The listing builds one solid part. Answer for the finished solid, in the listing's coordinates (mm). Face numbers are marked on the shaded views. Give positions to 0.01 mm unless a question says otherwise; leave off trailing zeros. Order: outer loops, then holes, each group sorted by start corner. A loop starts at its lowest first (then second) coordinate and runs counter-clockwise, first axis right, second up.
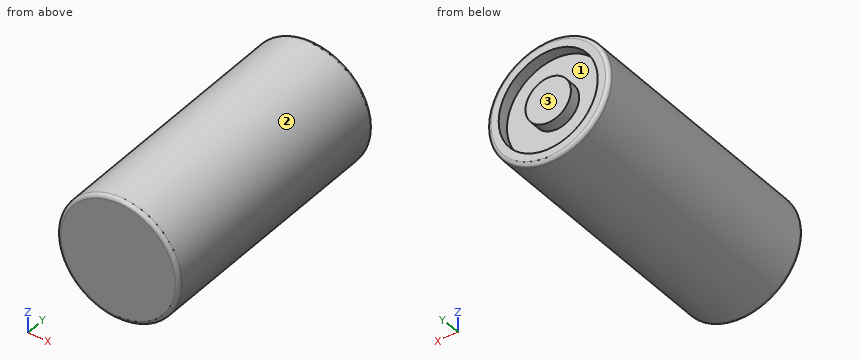
```python
from build123d import *

# Parameters (mm, degrees)
SKETCH_1_R          = 16.1
EXTRUDE_1_DEPTH     = 70.6
SKETCH_3_R          = 13.073776485
SKETCH_3_R_2        = 6
CUT_EXTRUDE_1_DEPTH = 3
FILLET_1_R          = 1
FILLET_2_R          = 1


with BuildPart() as part:
    # 草图1 → 凸台-拉伸1 (new body)
    with BuildSketch(Plane(origin=(0, 0, 0), x_dir=(1, 0, 0), z_dir=(0, 1, 0))):
        Circle(SKETCH_1_R)
    extrude(amount=EXTRUDE_1_DEPTH)

    # 草图3 → 切除-拉伸1 (cut)
    with BuildSketch(Plane(origin=(0, 70.6, 0), x_dir=(1, 0, 0), z_dir=(0, 1, 0))):
        Circle(SKETCH_3_R)
        Circle(SKETCH_3_R_2, mode=Mode.SUBTRACT)
    extrude(amount=-CUT_EXTRUDE_1_DEPTH, mode=Mode.SUBTRACT)

    # 圆角1
    fillet_1_edges = [part.edges().sort_by_distance(p)[0] for p in [
        (-16.1, 0, 0),
    ]]
    fillet(fillet_1_edges, radius=FILLET_1_R)

    # 圆角2
    fillet_2_edges = [part.edges().sort_by_distance(p)[0] for p in [
        (-16.1, 70.6, 0),
    ]]
    fillet(fillet_2_edges, radius=FILLET_2_R)


solid = part.part
```
1) Given P1, Ø8, axis at y = 58, z = -10.5, coming from the +X side; P2, Ø2, axis at y = 46.5, z = -4.5, coming from the -X side; P3, Ø10, axis at y = 50.5, z = -6, coming from the +X side, each flat-ended and moving along its own axis, determine where each tip first touches the part or whether it passes through.
Geometry says:
P1: stops at x = 14.73
P2: stops at x = -15.71
P3: stops at x = 16.07
2) Find section C-C (y = 60). Write down the section's boundary in (x, z), then the cut area to 3 significant figures.
Geometry says:
outline: circle Ø32.2 at (0, 0)
area: 814 mm2
3) Find section B-B (x = 0). Write down the section's boundary in (y, z), then the cut area to 3 significant figures.
Geometry says:
outline: (0, -15.1) arc R1 ccw to (1, -16.1) - (69.6, -16.1) arc R1 ccw to (70.6, -15.1) - (70.6, -13.07) - (67.6, -13.07) - (67.6, -6) - (70.6, -6) - (70.6, 6) - (67.6, 6) - (67.6, 13.07) - (70.6, 13.07) - (70.6, 15.1) arc R1 ccw to (69.6, 16.1) - (1, 16.1) arc R1 ccw to (0, 15.1) - close
area: 2,230 mm2
4) Straight lines are drawn through the part: probe 1 along Z at (x, y) = (0, 68.75); probe 2 along X at (y, z) = (70, 0). For each, find the intervals that lie inside material, in ascending order.
Geometry says:
probe 1: z = -16.1 to -13.07, -6 to 6, 13.07 to 16.1
probe 2: x = -16.02 to -13.07, -6 to 6, 13.07 to 16.02
5) Find section A-A (z = 0). Write down the section's boundary in (x, y), then the cut area to 3 significant figures.
Geometry says:
outline: (-16.1, 1) arc R1 ccw to (-15.1, 0) - (15.1, 0) arc R1 ccw to (16.1, 1) - (16.1, 69.6) arc R1 ccw to (15.1, 70.6) - (13.07, 70.6) - (13.07, 67.6) - (6, 67.6) - (6, 70.6) - (-6, 70.6) - (-6, 67.6) - (-13.07, 67.6) - (-13.07, 70.6) - (-15.1, 70.6) arc R1 ccw to (-16.1, 69.6) - close
area: 2,230 mm2
6) For a pull along X with two mould halves and no side action, classify the marked faces 1, 2 and 3 as +X half, -X half, draft (parallel to the pull), parting line (faces both ways), or undercut.
Geometry says:
face 1: undercut
face 2: parting line
face 3: draft
